```python
from build123d import *

# Parameters (mm, degrees)
F0_W     = 19.05
F0_H     = 19.05
F0_W_2   = 12.7
F0_H_2   = 12.7
F1_DEPTH = 114.3
F2_W     = 19.05
F2_H     = 19.05
F2_W_2   = 12.7
F2_H_2   = 12.7
F3_DEPTH = 63.5
F4_R     = 1.5875


with BuildPart() as f1:
    # F0 (on Front) → F1 (new body)
    with BuildSketch(Plane.XZ):
        with Locations((-80.5832530618, 119.2464818001)):
            Rectangle(F0_W, F0_H)
        with Locations((-80.5832530618, 119.2464818001)):
            Rectangle(F0_W_2, F0_H_2, mode=Mode.SUBTRACT)
    extrude(amount=-F1_DEPTH)

    # F2 (on face) → F3 (join)
    with BuildSketch(Plane.YZ.offset(-71.0582530618)):
        with Locations((57.15, 119.2464818001)):
            Rectangle(F2_W, F2_H)
        with Locations((57.15, 119.2464818001)):
            Rectangle(F2_W_2, F2_H_2, mode=Mode.SUBTRACT)
    extrude(amount=F3_DEPTH)

    # F4
    f4_edges = [f1.edges().sort_by_distance(p)[0] for p in [
        (-71.058253, 23.8125, 128.771482),
        (-39.308253, 47.625, 128.771482),
        (-90.108253, 57.15, 128.771482),
        (-71.058253, 23.8125, 109.721482),
        (-39.308253, 47.625, 109.721482),
        (-71.058253, 90.4875, 128.771482),
        (-71.058253, 90.4875, 109.721482),
        (-39.308253, 66.675, 109.721482),
        (-39.308253, 66.675, 128.771482),
        (-90.108253, 57.15, 109.721482),
    ]]
    fillet(f4_edges, radius=F4_R)


solid = f1.part
```
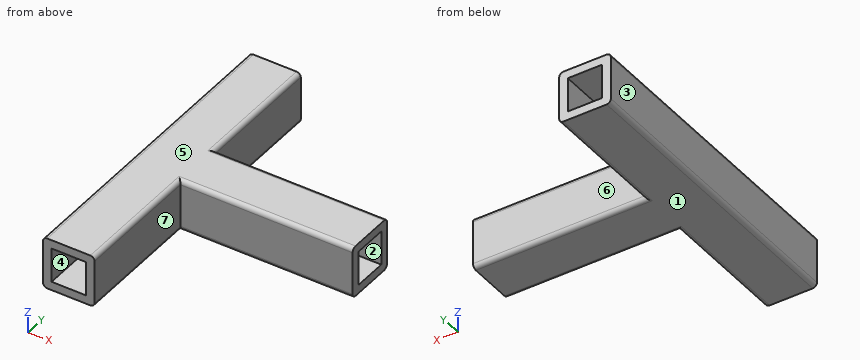
Can you work these out from the model? Positions are in its coordinate system, mm. Face numbers are marked on the shaded views. A direction names the side the tool comes from. Coordinates: 2 decimals unless noted, no trailing zeros. Loops run counter-clockwise (first coordinate to the right, second up) from the corner with the lowest first, then second, coordinate; pieces in that order, holes last. Notation, with made-up numbers: (43.25, 26.25) - (49.25, 26.25) arc R32 cw to (49.25, 62.25) - close; hole circle Ø7 at (29, -23.75). An arc over 180 degrees is marked (long way). Answer as CSV lines item,"result". Start each with the question number.
1) Suppose I cut it at C-C (x = -51.5). Please give me the cut outline in (y, z) (1 decimal).
2) Suppose I cut it at D-D (x = -77). Please give me the cut outline in (y, z), plus the area to 3 significant figures.
3) Suppose I cut it at B-B (y = 33). Please give me the cut outline in (x, z) (1 decimal).
4) Suppose I cut it at A-A (z = 115). Please give me the cut outline in (x, y) (3 decimals), plus the area to 3 significant figures.
5) Which directions (+Z, -Z, +X, -X, +Y, -Y) give clear straight access to the entire face, cutting with the end or side of a thin tool? Please do the marked faces 4, 5, 6 and 7.
6) Thinking about a two-plate mould opening in Z: for the marked faces 1, 2 and 3, which applies, pulls with the +Z half, pulls with the -Z half, needs draft (parallel to the pull), parting line crosses it, or undercut?
7) For pin 1 (4 mm diameter, centred on x = -34, z = 119, fed in from +Y) (3 decimals); pin 2 (1 mm diameter, centred on x = -25.5, z = 120.5, fed in from -Y) (3 decimals); pin 3 (10 mm diameter, centred on y = 57, z = 118.5, fed in from +X), each with a flat end and sliding along its axis, tell me the tip position at first contact or that it passes through.
8) I need wall thicknesses on line 1 (X direction, y = 62, z = 124.5); line 2 (Z direction, x = -75.5, y = 67.5); line 3 (X direction, y = 48.5, z = 123). Which ranges of each line are inside material? Lowest first, please. Write a range as from..to.
Check result:
1,outline,"(47.6, 111.3) arc R1.6 ccw to (49.2, 109.7) - (65.1, 109.7) arc R1.6 ccw to (66.7, 111.3) - (66.7, 127.2) arc R1.6 ccw to (65.1, 128.8) - (49.2, 128.8) arc R1.6 ccw to (47.6, 127.2) - close; hole (50.8, 112.9) - (63.5, 112.9) - (63.5, 125.6) - (50.8, 125.6) - close"
2,outline,"(0, 109.72) - (114.3, 109.72) - (114.3, 112.9) - (0, 112.9) - close; (0, 125.6) - (114.3, 125.6) - (114.3, 128.77) - (0, 128.77) - close"
2,area,"726 mm²"
3,outline,"(-90.1, 111.3) arc R1.6 ccw to (-88.5, 109.7) - (-72.6, 109.7) arc R1.6 ccw to (-71.1, 111.3) - (-71.1, 127.2) arc R1.6 ccw to (-72.6, 128.8) - (-88.5, 128.8) arc R1.6 ccw to (-90.1, 127.2) - close; hole (-86.9, 112.9) - (-74.2, 112.9) - (-74.2, 125.6) - (-86.9, 125.6) - close"
4,outline,"(-90.108, 0) - (-86.933, 0) - (-86.933, 114.3) - (-90.108, 114.3) - close; (-74.233, 0) - (-71.058, 0) - (-71.058, 47.625) - (-7.558, 47.625) - (-7.558, 50.8) - (-71.058, 50.8) - (-71.058, 63.5) - (-7.558, 63.5) - (-7.558, 66.675) - (-71.058, 66.675) - (-71.058, 114.3) - (-74.233, 114.3) - close"
4,area,"1,130 mm²"
5,face 4,"+Y, -Y"
5,face 5,"+Z, +X, -X, +Y, -Y"
5,face 6,"+Z, -Z, +X, +Y"
5,face 7,"+Z, -Z, +X, -Y"
6,face 1,"pulls with the -Z half"
6,face 2,"undercut"
6,face 3,"needs draft"
7,pin 1,"stops at y = 66.675"
7,pin 2,"stops at y = 47.625"
7,pin 3,"stops at x = -71.06"
8,line 1,"x = -90.11..-86.93, -74.23..-71.06"
8,line 2,"z = 109.72..112.9, 125.6..128.77"
8,line 3,"x = -90.11..-86.93, -74.23..-7.56"
